from build123d import *

# Parameters (mm, degrees)
F0_W     = 106.68
F0_H     = 152.4
F1_DEPTH = 3.175
F2_R     = 7.5
F3_DEPTH = 3.176


with BuildPart() as f1:
    # F0 (on Top) → F1 (new body)
    with BuildSketch(Plane.XY):
        Rectangle(F0_W, F0_H)
    extrude(amount=F1_DEPTH)

    # F2 (on face) → F3 (cut, through all)
    with BuildSketch(Plane.XY.offset(3.175)):
        with BuildLine():
            Line((-32.719586, -55.33588), (-38.523153, -60.20565))
            ThreePointArc((-38.523153, -60.20565), (-39.583374, -62.242316), (-38.892923, -64.432146))
            Line((-38.892923, -64.432146), (-35.427249, -68.562376))
            ThreePointArc((-35.427249, -68.562376), (-34.396971, -69.352936), (-33.129116, -69.634013))
            Line((-33.129116, -69.634013), (9.380051, -69.634013))
            ThreePointArc((9.380051, -69.634013), (10.406111, -69.453091), (11.308413, -68.932146))
            Line((11.308413, -68.932146), (17.11198, -64.062376))
            ThreePointArc((17.11198, -64.062376), (18.172201, -62.02571), (17.48175, -59.83588))
            Line((17.48175, -59.83588), (14.016076, -55.70565))
            ThreePointArc((14.016076, -55.70565), (12.985798, -54.91509), (11.717943, -54.634013))
            Line((11.717943, -54.634013), (-30.791223, -54.634013))
            ThreePointArc((-30.791223, -54.634013), (-31.817284, -54.814935), (-32.719586, -55.33588))
        make_face()
        with BuildLine():
            ThreePointArc((-44.035224, -58.303791), (-41.998558, -59.364012), (-39.808728, -58.673561))
            Line((-39.808728, -58.673561), (-34.005161, -53.803791))
            ThreePointArc((-34.005161, -53.803791), (-33.335448, -53.005657), (-32.979101, -52.026602))
            Line((-32.979101, -52.026602), (-25.597462, -10.163245))
            ThreePointArc((-25.597462, -10.163245), (-25.654107, -8.865844), (-26.253752, -7.713938))
            Line((-26.253752, -7.713938), (-29.719426, -3.583709))
            ThreePointArc((-29.719426, -3.583709), (-31.756092, -2.523487), (-33.945922, -3.213938))
            Line((-33.945922, -3.213938), (-39.749488, -8.083709))
            ThreePointArc((-39.749488, -8.083709), (-40.419202, -8.881842), (-40.775549, -9.860897))
            Line((-40.775549, -9.860897), (-48.157188, -51.724254))
            ThreePointArc((-48.157188, -51.724254), (-48.100542, -53.021656), (-47.500898, -54.173561))
            Line((-47.500898, -54.173561), (-44.035224, -58.303791))
        make_face()
        with BuildLine():
            ThreePointArc((14.891875, -51.970768), (14.948521, -53.268169), (15.548165, -54.420075))
            Line((15.548165, -54.420075), (19.013839, -58.550304))
            ThreePointArc((19.013839, -58.550304), (21.050505, -59.610526), (23.240335, -58.920075))
            Line((23.240335, -58.920075), (29.043902, -54.050304))
            ThreePointArc((29.043902, -54.050304), (29.713615, -53.252171), (30.069962, -52.273116))
            Line((30.069962, -52.273116), (37.451602, -10.409759))
            ThreePointArc((37.451602, -10.409759), (37.394956, -9.112357), (36.795312, -7.960452))
            Line((36.795312, -7.960452), (33.329638, -3.830222))
            ThreePointArc((33.329638, -3.830222), (31.292972, -2.770001), (29.103141, -3.460452))
            Line((29.103141, -3.460452), (23.299575, -8.330222))
            ThreePointArc((23.299575, -8.330222), (22.629862, -9.128356), (22.273515, -10.107411))
            Line((22.273515, -10.107411), (14.891875, -51.970768))
        make_face()
        with BuildLine():
            ThreePointArc((-27.817566, 1.928363), (-28.877788, -0.108303), (-28.187337, -2.298133))
            Line((-28.187337, -2.298133), (-24.721663, -6.428363))
            ThreePointArc((-24.721663, -6.428363), (-23.691384, -7.218923), (-22.423529, -7.5))
            Line((-22.423529, -7.5), (20.085637, -7.5))
            ThreePointArc((20.085637, -7.5), (21.111697, -7.319078), (22.014, -6.798133))
            Line((22.014, -6.798133), (27.817566, -1.928363))
            ThreePointArc((27.817566, -1.928363), (28.877788, 0.108303), (28.187337, 2.298133))
            Line((28.187337, 2.298133), (24.721663, 6.428363))
            ThreePointArc((24.721663, 6.428363), (23.691384, 7.218923), (22.423529, 7.5))
            Line((22.423529, 7.5), (-20.085637, 7.5))
            ThreePointArc((-20.085637, 7.5), (-21.111697, 7.319078), (-22.014, 6.798133))
            Line((-22.014, 6.798133), (-27.817566, 1.928363))
        make_face()
        with BuildLine():
            ThreePointArc((-33.329638, 3.830222), (-31.292972, 2.770001), (-29.103141, 3.460452))
            Line((-29.103141, 3.460452), (-23.299575, 8.330222))
            ThreePointArc((-23.299575, 8.330222), (-22.629862, 9.128356), (-22.273515, 10.107411))
            Line((-22.273515, 10.107411), (-14.891875, 51.970768))
            ThreePointArc((-14.891875, 51.970768), (-14.948521, 53.268169), (-15.548165, 54.420075))
            Line((-15.548165, 54.420075), (-19.013839, 58.550304))
            ThreePointArc((-19.013839, 58.550304), (-21.050505, 59.610526), (-23.240335, 58.920075))
            Line((-23.240335, 58.920075), (-29.043902, 54.050304))
            ThreePointArc((-29.043902, 54.050304), (-29.713615, 53.252171), (-30.069962, 52.273116))
            Line((-30.069962, 52.273116), (-37.451602, 10.409759))
            ThreePointArc((-37.451602, 10.409759), (-37.394956, 9.112357), (-36.795312, 7.960452))
            Line((-36.795312, 7.960452), (-33.329638, 3.830222))
        make_face()
        with BuildLine():
            ThreePointArc((25.597462, 10.163245), (25.654107, 8.865844), (26.253752, 7.713938))
            Line((26.253752, 7.713938), (29.719426, 3.583709))
            ThreePointArc((29.719426, 3.583709), (31.756092, 2.523487), (33.945922, 3.213938))
            Line((33.945922, 3.213938), (39.749488, 8.083709))
            ThreePointArc((39.749488, 8.083709), (40.419202, 8.881842), (40.775549, 9.860897))
            Line((40.775549, 9.860897), (48.157188, 51.724254))
            ThreePointArc((48.157188, 51.724254), (48.100542, 53.021656), (47.500898, 54.173561))
            Line((47.500898, 54.173561), (44.035224, 58.303791))
            ThreePointArc((44.035224, 58.303791), (41.998558, 59.364012), (39.808728, 58.673561))
            Line((39.808728, 58.673561), (34.005161, 53.803791))
            ThreePointArc((34.005161, 53.803791), (33.335448, 53.005657), (32.979101, 52.026602))
            Line((32.979101, 52.026602), (25.597462, 10.163245))
        make_face()
        with BuildLine():
            ThreePointArc((-17.11198, 64.062376), (-18.172201, 62.02571), (-17.48175, 59.83588))
            Line((-17.48175, 59.83588), (-14.016076, 55.70565))
            ThreePointArc((-14.016076, 55.70565), (-12.985798, 54.91509), (-11.717943, 54.634013))
            Line((-11.717943, 54.634013), (30.791223, 54.634013))
            ThreePointArc((30.791223, 54.634013), (31.817284, 54.814935), (32.719586, 55.33588))
            Line((32.719586, 55.33588), (38.523153, 60.20565))
            ThreePointArc((38.523153, 60.20565), (39.583374, 62.242316), (38.892923, 64.432146))
            Line((38.892923, 64.432146), (35.427249, 68.562376))
            ThreePointArc((35.427249, 68.562376), (34.396971, 69.352936), (33.129116, 69.634013))
            Line((33.129116, 69.634013), (-9.380051, 69.634013))
            ThreePointArc((-9.380051, 69.634013), (-10.406111, 69.453091), (-11.308413, 68.932146))
            Line((-11.308413, 68.932146), (-17.11198, 64.062376))
        make_face()
        with Locations((44.880354, -45.848438)):
            Circle(F2_R)
    extrude(amount=-F3_DEPTH, mode=Mode.SUBTRACT)


solid = f1.part
The listing builds one solid part. Answer for the finished solid, in the listing's coordinates (mm). A direction names the side the tool comes from. Coordinates: 2 decimals unless noted, no trailing zeros. Order: outer loops, then holes, each group sorted by start corner. A loop starts at its lowest first (then second) coordinate and runs counter-clockwise, first axis right, second up.
Q1. A cutting plane is placed at D-D, the plane z = 0.75. State how many separate pieces and enclosed holes the cut face has, and give its area (3 significant figures).
Q2. Which of the six approach directions +Z, -Z, +X, -X, +Y, -Y give full straight-line access (tool end or side, diameter ignored) to faces 3 (the face through (45.8, 56.2, 1.6)), 4 (the face through (-53.34, -1, 2))?
Q3. Given P1, Ø9, axis at x = 44.88, y = -45.85, coming from the -Z side, flat-ended and moving along its own axis, determine where the tip first touches the part or whether it passes through.
Q4. A cutting plane is placed at C-C, the plane y = 45. Write down the section's boundary in (x, z) (3 decimals), and give its area (3 significant figures).
Q5. A cutting plane is placed at A-A, the plane x = 4.5. Write down the section's boundary in (y, z) (3 decimals).
Q6. A cutting plane is placed at B-B, the plane y = 62. Write down the section's boundary in (x, z) (3 decimals), and give its area (3 significant figures).
Q7. For a pull along Y with two mould halves and no side action, classify faces 1 (the face through (1, 7.5, 2)), 2 (the face through (-1, 18, 0)) as pulls with the +Y half, pulls with the -Y half, needs draft (parallel to the pull), parting line crosses it, or undercut.
Q8. Consider line 1 (Y direction, x = -4, z = 1.25); line 2 (Y direction, x = 22.5, z = 1.6); line 3 (X direction, y = 59, z = 0.35). Determine where each line is inside the solid, lowest interval first.
Answers follow:
1. separate pieces: 1
1. enclosed holes: 8
1. area: 10,600 mm2
2. face 3: +Z, -Z
2. face 4: +Z, -Z, -X, +Y, -Y
3. P1: passes through
4. outline: (-53.34, 0) - (-31.352, 0) - (-31.352, 3.175) - (-53.34, 3.175) - close; (-16.121, 0) - (31.74, 0) - (31.74, 3.175) - (-16.121, 3.175) - close; (46.972, 0) - (53.34, 0) - (53.34, 3.175) - (46.972, 3.175) - close
4. area: 242 mm2
5. outline: (-76.2, 0) - (-69.634, 0) - (-69.634, 3.175) - (-76.2, 3.175) - close; (-54.634, 0) - (-7.5, 0) - (-7.5, 3.175) - (-54.634, 3.175) - close; (7.5, 0) - (54.634, 0) - (54.634, 3.175) - (7.5, 3.175) - close; (69.634, 0) - (76.2, 0) - (76.2, 3.175) - (69.634, 3.175) - close
6. outline: (-53.34, 0) - (-18.174, 0) - (-18.174, 3.175) - (-53.34, 3.175) - close; (39.552, 0) - (53.34, 0) - (53.34, 3.175) - (39.552, 3.175) - close
6. area: 155 mm2
7. face 1: undercut
7. face 2: needs draft
8. line 1: y = -76.2 to -69.63, -54.63 to -7.5, 7.5 to 54.63, 69.63 to 76.2
8. line 2: y = -76.2 to -59.38, -9.38 to -6.39, 7.5 to 54.63, 69.63 to 76.2
8. line 3: x = -53.34 to -23.14, -19.48 to -16.78, 37.09 to 40.28, 43.19 to 53.34
